from build123d import *

# Parameters (mm, degrees)
EXTRUDE_START       = -10.064513
EXTRUDE_1_DEPTH     = 40.064513032
SKETCH_2_R          = 5.499999999
CUT_EXTRUDE_2_DEPTH = 5.5
SKETCH_3_R          = 1.999999999
CUT_EXTRUDE_3_DEPTH = 4


with BuildPart() as part:
    # Эскиз1 → Вытянуть1 (new body)
    with BuildSketch(Plane.XY.offset(EXTRUDE_START)):
        with BuildLine():
            Line((-10.958966345, 5.977749985), (10.958966345, 5.977749985))
            Line((10.958966345, 5.977749985), (10.958966345, -4.027821729))
            ThreePointArc((10.958966345, -4.027821729), (9.072657082, -5.563138372), (7.432238503, -7.358796112))
            Line((7.432238503, -7.358796112), (-7.432238503, -7.358796112))
            ThreePointArc((-7.432238503, -7.358796112), (-9.072657082, -5.563138372), (-10.958966345, -4.027821729))
            Line((-10.958966345, -4.027821729), (-10.958966345, 5.977749985))
        make_face()
    extrude(amount=EXTRUDE_1_DEPTH)

    # Эскиз2 → Вытянуть2 (cut)
    with BuildSketch(Plane.XZ.offset(7.358796112)):
        with Locations(Location((0, 9.967743485, 0), (0, 0, 270))):
            Circle(SKETCH_2_R)
    extrude(amount=-CUT_EXTRUDE_2_DEPTH, mode=Mode.SUBTRACT)

    # Эскиз3 → Вытянуть3 (cut)
    with BuildSketch(Plane.XZ.offset(1.858796112)):
        with Locations(Location((0, 9.967743485, 0), (0, 0, 270))):
            Circle(SKETCH_3_R)
    extrude(amount=-CUT_EXTRUDE_3_DEPTH, mode=Mode.SUBTRACT)


solid = part.part
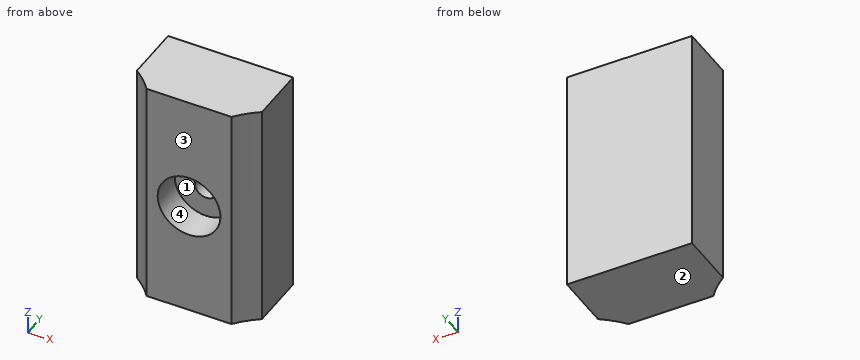
Part model, mm, in its own coordinate system. Face numbers are marked on the shaded views. Round coordinates to 2 decimals unless told otherwise and drop trailing zeros. Write each loop counter-clockwise with the first axis right and the second up, starting at its lowest first coordinate (ties: lowest second). Pieces come first, ordered by that corner, then holes. Notation, with made-up numbers: M 69.25,34.5 L 88.25,34.5 A31 ccw 88.25,70.5 Z; hole C -21.75,-16 d1. An arc over 180 degrees is marked long. Return JSON: item names as keys, results as strings. Group by question number.
(1) Saw through at D-D on x = 3. Write the cut outline in (y, z), then the cut area to 3 significant figures.
(2) Saw through at A-A on x = 0. Write the cut outline in (y, z).
(3) Two-plate mould, pull along Z, no slides. Class the marked faces 1, 2, 3 and 4: +Z half, -Z half, draft (parallel to the pull), parting line (faces both ways), or undercut.
(4) Saw through at C-C on z = 8.5. Write the cut outline in (x, y), then the cut area to 3 significant figures.
(5) Drill centre lines: probe 1 along Z at (x, y) = (4.5, -4.25); probe 2 along Z at (x, y) = (5, -2.25); probe 3 along X at (y, z) = (-2, 12.5). Where is each one in solid material? Low to high.
(6) Saw through at B-B on z = 26. Write the cut outline in (x, y), then the cut area to 3 significant figures.
(7) Pin check, flat tip, straight feed: pin 1 Ø3 at (x, z) = (0.5, 11) entering from -Y. Stop position of the tip, or through.
Returned:
{
 "1": {"outline": "M -7.36,-10.06 L 5.98,-10.06 L 5.98,30 L -7.36,30 L -7.36,14.58 L -1.86,14.58 L -1.86,5.36 L -7.36,5.36 Z", "area": "484 mm²"},
 "2": {"outline": "M -7.36,-10.06 L 5.98,-10.06 L 5.98,30 L -7.36,30 L -7.36,15.47 L -1.86,15.47 L -1.86,11.97 L 2.14,11.97 L 2.14,7.97 L -1.86,7.97 L -1.86,4.47 L -7.36,4.47 Z"},
 "3": {"face 1": "undercut", "face 2": "-Z half", "face 3": "draft", "face 4": "undercut"},
 "4": {"outline": "M -10.96,-4.03 A16.52 cw -7.43,-7.36 L -5.3,-7.36 L -5.3,-1.86 L -1.36,-1.86 L -1.36,2.14 L 1.36,2.14 L 1.36,-1.86 L 5.3,-1.86 L 5.3,-7.36 L 7.43,-7.36 A16.52 cw 10.96,-4.03 L 10.96,5.98 L -10.96,5.98 Z", "area": "210 mm²"},
 "5": {"probe 1": "-10.06 to 6.81, 13.13 to 30", "probe 2": "-10.06 to 7.68, 12.26 to 30", "probe 3": "-10.96 to -4.88, 4.88 to 10.96"},
 "6": {"outline": "M -10.96,-4.03 A16.52 cw -7.43,-7.36 L 7.43,-7.36 A16.52 cw 10.96,-4.03 L 10.96,5.98 L -10.96,5.98 Z", "area": "279 mm²"},
 "7": {"pin 1": "y = -1.86"}
}
